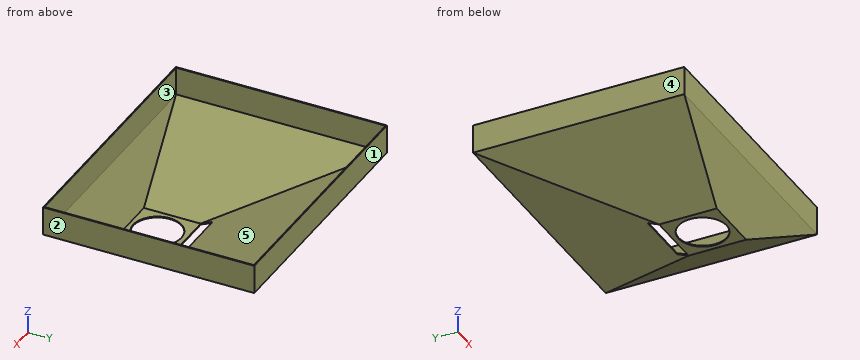
from build123d import *

# Parameters (mm, degrees)
EXTRUDE_1_REACH     = 237
SKETCH_7_W          = 270
SKETCH_7_H          = 220
SHELL_1_T           = -1
SKETCH_8_R          = 25
CUT_EXTRUDE_2_DEPTH = 10
SKETCH_9_W          = 60
SKETCH_9_H          = 12
CUT_EXTRUDE_3_DEPTH = 10


with BuildPart() as part:
    # 草图2 → 放样1 section 0
    with BuildSketch(Plane.XY.offset(60)):
        with BuildLine():
            Line((-135, 170), (135, 170))
            Line((135, 170), (135, -50))
            Line((135, -50), (-135, -50))
            Line((-135, -50), (-135, 170))
        make_face()
    # 草图1 → 放样1 section 1
    with BuildSketch(Plane.XY):
        with BuildLine():
            Line((-30, 30), (30, 30))
            Line((30, 30), (30, -30))
            Line((30, -30), (-30, -30))
            Line((-30, -30), (-30, 30))
        make_face()
    loft()

    # 草图7 → 凸台-拉伸1 (add, up to next)
    with BuildSketch(Plane.XY.offset(90), mode=Mode.PRIVATE) as extrude_1_sk1:
        with Locations((0, 60)):
            Rectangle(SKETCH_7_W, SKETCH_7_H)
    extrude_1_tool1 = extrude(extrude_1_sk1.sketch, amount=-EXTRUDE_1_REACH, mode=Mode.PRIVATE) - part.part
    add(extrude_1_tool1.solids().sort_by_distance((0, 60, 90))[0])

    # 抽壳1
    shell_1_openings = [part.faces().sort_by_distance(p)[0] for p in [
        (0, 60, 90),
    ]]
    offset(amount=SHELL_1_T, openings=shell_1_openings)

    # 草图8 → 切除-拉伸2 (cut)
    with BuildSketch(Plane.XY.offset(1)):
        Circle(SKETCH_8_R)
    extrude(amount=-CUT_EXTRUDE_2_DEPTH, mode=Mode.SUBTRACT)

    # 草图9 → 切除-拉伸3 (cut)
    with BuildSketch(Plane(origin=(0, 0, 0), x_dir=(-1, 0, 0), z_dir=(0, 0, -1))):
        with Locations((0, 36)):
            Rectangle(SKETCH_9_W, SKETCH_9_H)
    extrude(amount=-CUT_EXTRUDE_3_DEPTH, mode=Mode.SUBTRACT)


solid = part.part
Work out the finished part from the listing and answer in its coordinate system (mm). Face numbers are marked on the shaded views. A direction names the side the tool comes from. Give positions to 0.01 mm unless a question says otherwise; leave off trailing zeros. One line per item, written item: value.
Item 1: Find section A-A, the plane x = 0. State how many separate pieces and enclosed holes the cut face has, plus the area to 3 significant figures.
Answer sheet:
separate pieces: 3
enclosed holes: 0
area: 271 mm²
Item 2: A tool of negligible diameter and unlimited length cuts with its end or side. For the marked faces 4 and 5, from which of +Z, -Z, +X, -X, +Y, -Y can it reach the whole face along a straight path? Write none if from no direction.
Answer sheet:
face 4: +Z, -Z, -X, +Y, -Y
face 5: +Z
Item 3: Determine the mould class of the marked faces 1, 2 and 3 for opening direction X: released by +X, released by -X, zero draft, split by the parting line, or undercut.
Answer sheet:
face 1: zero draft
face 2: released by +X
face 3: undercut
Item 4: Flat-ended cylindrical pins translate along their axes: P1, Ø5, axis at y = 37.5, z = 1.5, coming from the +X side; P2, Ø8, axis at y = 129, z = 49.5, coming from the +X side (3 decimals); P3, Ø8, axis at x = 52, y = 23, coming from the +Z side; P4, Ø10, axis at y = 23.5, z = 59.5, coming from the +X side. Find the tip coordinate at first contact, or state that the pin passes through.
Answer sheet:
P1: x = 37
P2: x = 123.625
P3: z = 16.01
P4: x = 135
Item 5: Straight lines are drawn through the part: probe 1 along X at (y, z) = (25, 80); probe 2 along Y at (x, z) = (-97.5, 62.5); probe 3 along X at (y, z) = (58, 55). For each, find the intervals that lie inside material, in ascending order.
Answer sheet:
probe 1: -135 to -134, 134 to 135
probe 2: -50 to -49, 169 to 170
probe 3: -126.25 to -124.23, 124.23 to 126.25
